The listing builds one solid part. Answer for the finished solid, in the listing's coordinates (mm). Face numbers are marked on the shaded views. A direction names the side the tool comes from. Round coordinates to 2 decimals unless told otherwise and drop trailing zeros. Write each loop counter-clockwise with the first axis right and the second up, starting at its lowest first coordinate (ties: lowest second). Pieces come first, ordered by that corner, then holes.
(1) A cutting plane is placed at C-C, the plane y = 34.5. Give the vertices of the cut face in (x, z).
(2) The mould has two halves that part along X. Classify the marked faces 1, 2, 3 and 4: +X half, -X half, draft (parallel to the pull), parting line (faces both ways), or undercut.
(3) A cutting plane is placed at D-D, the plane z = 36.5. Give the vertices of the cut face in (x, y).
(4) Find the intervals of material crossed by probe 1 along Y at (x, z) = (4, 76); probe 2 along Y at (x, z) = (101.75, 6.35); probe 3 along X at (y, z) = (69, 18.5), in increasing order.
(5) A cutting plane is placed at A-A, the plane y = 12.7. Give the vertices of the cut face in (x, z).
(6) For the marked faces 5, 6 and 7, determine the directions among +Z, -Z, +X, -X, +Y, -Y from which every point of the face is accessible in a straight line to the end or side of a thin tool.
(7) Each of these flat-tipped pins is pushed along its axis until it touches: pin 1 Ø2 at (x, z) = (57.5, 26) entering from +Y; pin 2 Ø4.5 at (y, z) = (12.7, 76.2) entering from +X; pin 3 Ø2 at (x, z) = (25.5, 42) entering from -Y; pin 4 Ø4 at (y, z) = (87, 74) entering from +X. Where does it stop, or does it pass through?
(8) A cutting plane is placed at B-B, the plane z = 76.2. Give the number of separate pieces and of enclosed holes in the cut face, and give its area (3 significant figures).
from build123d import *

# Parameters (mm, degrees)
SKETCH1_W                   = 25.4
SKETCH1_H                   = 25.4
SKETCH1_R                   = 6.35
BOSS_EXTRUDE1_DEPTH         = 82.55
FILLET1_R                   = 6.35
SKETCH3_W                   = 136.608571953
SKETCH3_H                   = 27.79521791
SKETCH3_H_2                 = 56.261
SKETCH3_H_3                 = 24.259466636
CUT_EXTRUDE3_DEPTH          = 31.75
TAP_DRILL_FOR_1_4_20_TAP1_D = 5.1054


with BuildPart() as part:
    # Sketch1 → Boss-Extrude1 (new body)
    # profile 1 of 2: a face of its own
    with BuildSketch(Plane.XY):
        with Locations((52.451, 89.662)):
            Rectangle(SKETCH1_W, SKETCH1_H)
        with Locations((52.451, 92.837)):
            Circle(SKETCH1_R, mode=Mode.SUBTRACT)
    # profile 2 of 2: a face of its own
    with BuildSketch(Plane.XY):
        Polygon((6.35, 70.612), (98.552, 70.612), (98.552, 0), (104.902, 0), (104.902, 76.962), (0, 76.962), (0, 0), (6.35, 0), align=None)
    extrude(amount=BOSS_EXTRUDE1_DEPTH)

    # Fillet1
    fillet1_edges = [part.edges().sort_by_distance(p)[0] for p in [
        (65.151, 76.962, 41.275),
        (39.751, 76.962, 41.275),
        (39.751, 102.362, 41.275),
        (65.151, 102.362, 41.275),
    ]]
    fillet(fillet1_edges, radius=FILLET1_R)

    # Sketch3 → Cut-Extrude3 (cut)
    with BuildSketch(Plane(origin=(0, 108.712, 0), x_dir=(1, 0, 0), z_dir=(0, 1, 0))):
        with Locations((56.578258919, 13.453108955)):
            Rectangle(SKETCH3_W, SKETCH3_H)
        with Locations((56.578258919, -41.275)):
            Rectangle(SKETCH3_W, SKETCH3_H_2)
        with Locations((56.578258919, -94.235233318)):
            Rectangle(SKETCH3_W, SKETCH3_H_3)
    extrude(amount=-CUT_EXTRUDE3_DEPTH, mode=Mode.SUBTRACT)

    # Tap Drill for 1/4-20 Tap1 (through all)
    with Locations(Plane.ZY):
        with Locations((6.35, 50.8), (6.35, 12.7), (76.2, 12.7), (76.2, 50.8)):
            Hole(TAP_DRILL_FOR_1_4_20_TAP1_D / 2)


solid = part.part
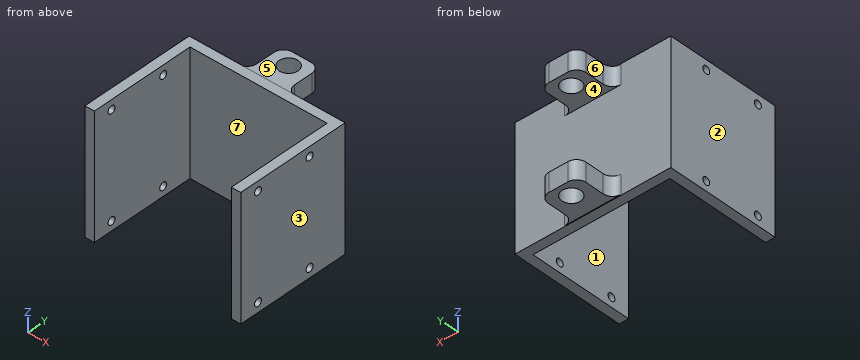
Solutions:
1. outline: (0, 0) - (6.35, 0) - (6.35, 82.55) - (0, 82.55) - close; (98.55, 0) - (104.9, 0) - (104.9, 82.55) - (98.55, 82.55) - close
2. face 1: undercut
2. face 2: -X half
2. face 3: +X half
2. face 4: draft
3. outline: (0, 0) - (6.35, 0) - (6.35, 70.61) - (98.55, 70.61) - (98.55, 0) - (104.9, 0) - (104.9, 76.96) - (0, 76.96) - close
4. probe 1: y = 0 to 10.16, 15.24 to 48.26, 53.34 to 76.96
4. probe 2: y = 0 to 10.15, 15.25 to 48.25, 53.35 to 76.96
4. probe 3: x = 0 to 6.35, 98.55 to 104.9
5. outline: (0, 0) - (6.35, 0) - (6.35, 3.8) - (0, 3.8) - close; (0, 8.9) - (6.35, 8.9) - (6.35, 73.65) - (0, 73.65) - close; (0, 78.75) - (6.35, 78.75) - (6.35, 82.55) - (0, 82.55) - close; (98.55, 0) - (104.9, 0) - (104.9, 3.8) - (98.55, 3.8) - close; (98.55, 8.9) - (104.9, 8.9) - (104.9, 73.65) - (98.55, 73.65) - close; (98.55, 78.75) - (104.9, 78.75) - (104.9, 82.55) - (98.55, 82.55) - close
6. face 5: +Z, +X, -X, +Y
6. face 6: +Z, -Z, -X, +Y
6. face 7: +Z, -Z, -Y
7. pin 1: stops at y = 76.96
7. pin 2: passes through
7. pin 3: stops at y = 70.61
7. pin 4: stops at x = 65.15
8. separate pieces: 5
8. enclosed holes: 1
8. area: 1,950 mm2
